Autodesk Inventor part; units mm, degrees
ref_plane "YZ Plane" through (0, 0, 0) normal (1, 0, 0) x (0, 1, 0)
ref_plane "XZ Plane" through (0, 0, 0) normal (0, 1, 0) x (-1, 0, 0)
ref_plane "XY Plane" through (0, 0, 0) normal (0, 0, 1) x (1, 0, 0)
sketch "Sketch1" plane through (0, 0, 0) normal (0, 0, 1) x (1, 0, 0)
  line L0 (-28.575, -19.685) -> (28.575, -19.685)
  line L1 (28.575, -19.685) -> (28.575, 19.685)
  line L2 (28.575, 19.685) -> (-28.575, 19.685)
  line L3 (-28.575, 19.685) -> (-28.575, -19.685)
  line L4 (-28.575, -19.685) -> (28.575, 19.685) construction
  line L5 (28.575, -19.685) -> (-28.575, 19.685) construction
  line L6 (-30.353, 21.463) -> (30.353, 21.463)
  line L7 (30.353, 21.463) -> (30.353, -21.463)
  line L8 (30.353, -21.463) -> (-30.353, -21.463)
  line L9 (-30.353, -21.463) -> (-30.353, 21.463)
  point P0 (0, 0)
  dimension "d0" = 57.15
  dimension "d1" = 39.37
  dimension "d2" = 1.778
extrude "Extrusion1" add sketch "Sketch1" along normal mid plane 1.778
fillet "Fillet1" radius 1 4 edges at (-28.575, -19.685, 0) (-28.575, 19.685, 0) (28.575, 19.685, 0) (28.575, -19.685, 0)
fillet "Fillet1" radius 1.5 4 edges at (-30.353, 21.463, 0) (-30.353, -21.463, 0) (30.353, -21.463, 0) (30.353, 21.463, 0)
properties part number "O-RING DASH 036 SQUARE"
Model file for the job. Use its own axes, mm. A direction names the side the tool comes from. Give positions to 0.01 mm unless a question says otherwise; leave off trailing zeros. Loops run counter-clockwise (first coordinate to the right, second up) from the corner with the lowest first, then second, coordinate; pieces in that order, holes last. Notation, with made-up numbers: M 58.5,55.25 L 84.5,55.25 A22 ccw 84.5,66.25 Z; hole C 40,6.25 d2. An arc over 180 degrees is marked long. Use one line per item in the form item = value.
Item 1: Which spindle directions (+Z, -Z, +X, -X, +Y, -Y) get a long thin tool onto all of the face, cutting with end or side? Do faces 1 (the cylindrical face through (29.925, -21.012, -0.012)), 2 (the flat face through (28.575, 0, 0)). Say none if no direction does.
Filled in:
face_1 = +Z, -Z, +X, -Y
face_2 = +Z, -Z
Item 2: Flat gauge pin, fed straight in: pin 1 Ø12 at (x, y) = (18, 1.5) entering from -Z. Where does the tip first touch, or does it go through?
Filled in:
pin_1 = through
Item 3: Two-plate mould, pull along Y, no slides. Class faces 3 (the flat face through (-2, -21, 0.889)), 4 (the flat face through (0, 19.685, 0)), 5 (the flat face through (0, 21.463, 0)), 6 (the flat face through (0, -21.463, 0)): released by +Y, released by -Y, zero draft, split by the parting line, or undercut.
Filled in:
face_3 = zero draft
face_4 = undercut
face_5 = released by +Y
face_6 = released by -Y
Item 4: Slice it at A-A on y = -16. List the corners of the cut face in (x, z) (3 decimals), and give its area (3 significant figures).
Filled in:
outline = M -30.353,-0.889 L -28.575,-0.889 L -28.575,0.889 L -30.353,0.889 Z; M 28.575,-0.889 L 30.353,-0.889 L 30.353,0.889 L 28.575,0.889 Z
area = 6.32 mm^2
Item 5: Slice it at B-B on z = -0.5. List the corners of the cut face in (x, y) (3 decimals), and give its area (3 significant figures).
Filled in:
outline = M -30.353,-19.963 A1.5 ccw -28.853,-21.463 L 28.853,-21.463 A1.5 ccw 30.353,-19.963 L 30.353,19.963 A1.5 ccw 28.853,21.463 L -28.853,21.463 A1.5 ccw -30.353,19.963 Z; hole M -28.575,-18.685 A1 ccw -27.575,-19.685 L 27.575,-19.685 A1 ccw 28.575,-18.685 L 28.575,18.685 A1 ccw 27.575,19.685 L -27.575,19.685 A1 ccw -28.575,18.685 Z
area = 355 mm^2
Item 6: Slice it at C-C on x = -19. List the corners of the cut face in (y, z) (3 decimals), and give its area (3 significant figures).
Filled in:
outline = M -21.463,-0.889 L -19.685,-0.889 L -19.685,0.889 L -21.463,0.889 Z; M 19.685,-0.889 L 21.463,-0.889 L 21.463,0.889 L 19.685,0.889 Z
area = 6.32 mm^2
Item 7: Drill centre lines: L1, parallel to X at y = -10, z = -0.55 (3 decimals); L2, parallel to Y at x = 4.5, z = -0.5 (3 decimals); L3, parallel to X at y = 19, z = -0.25. Where is each one in solid material? Low to high.
Filled in:
L1 = -30.353 to -28.575, 28.575 to 30.353
L2 = -21.463 to -19.685, 19.685 to 21.463
L3 = -30.35 to -28.52, 28.52 to 30.35
